Here's the drawing with two shaded views (mm, measured from the low corner). I have some questions. Coordinates: 2 decimals unless noted, no trailing zeros. Order: outer loops, then holes, each group sorted by start corner. A loop starts at its lowest first (then second) coordinate and runs counter-clockwise, first axis right, second up. Notation, with made-up numbers: (-19.75, -15.75) -> (-5.75, -15.75) arc R26 cw to (-5.75, 17.25) -> close; hole circle Ø5 at (74, 3.5). An arc over 180 degrees is marked (long way). Write item = value, one per line.
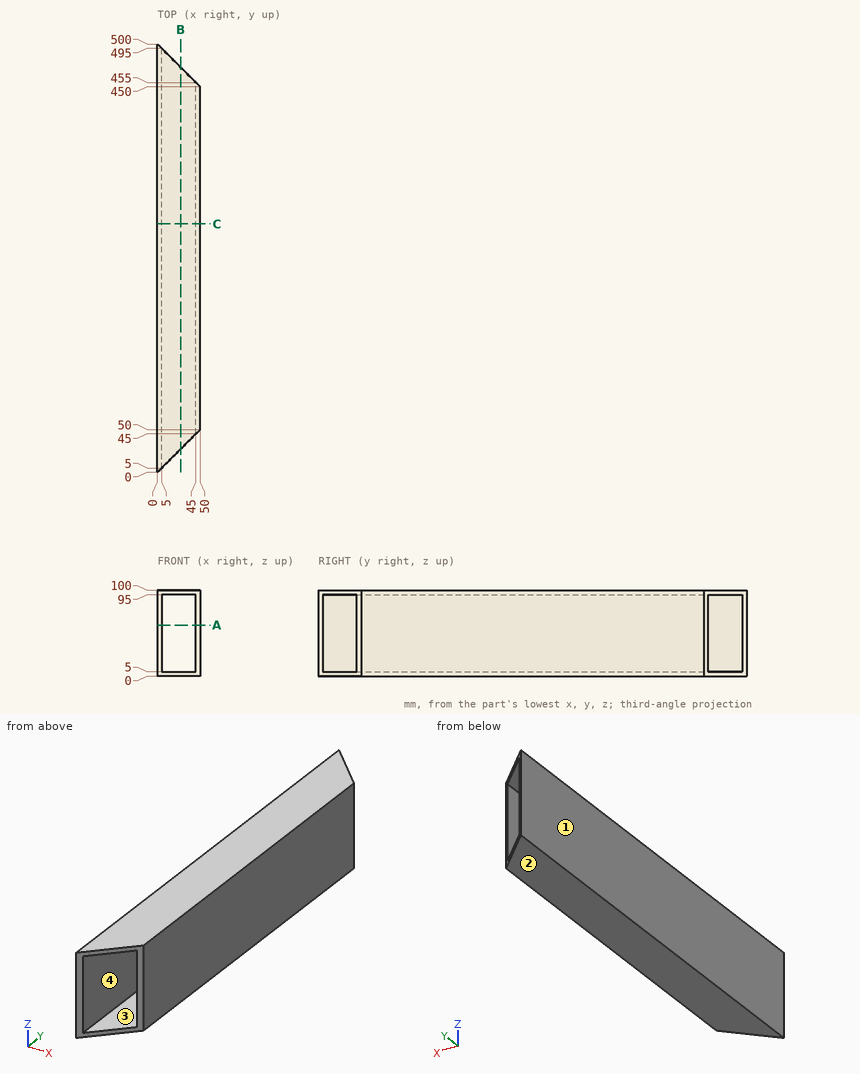
Item 1: I want a section at B-B, the plane x = 27. Please give me the cut outline in (y, z).
A:
outline = (27, 0) -> (473, 0) -> (473, 5) -> (27, 5) -> close; (27, 95) -> (473, 95) -> (473, 100) -> (27, 100) -> close
Item 2: I want a section at C-C, the plane y = 290. Please give me the cut outline in (x, z).
A:
outline = (0, 0) -> (50, 0) -> (50, 100) -> (0, 100) -> close; hole (5, 5) -> (45, 5) -> (45, 95) -> (5, 95) -> close
Item 3: I'm going to push flat-ended pins straight in: P1, Ø5, axis at x = 14, y = 93, coming from the -Z side; P2, Ø6, axis at x = 7.5, z = 54, coming from the -Y side. Where does each tip first touch, or does it pass through?
A:
P1 = 0
P2 = 4.5
Item 4: If we mould it in two halves opening along X, with no side actions, what happens to the marked faces 1, 2, 3 and 4? For each: pulls with the +X half, pulls with the -X half, needs draft (parallel to the pull), parting line crosses it, or undercut.
A:
face_1 = pulls with the -X half
face_2 = needs draft
face_3 = undercut
face_4 = undercut
Item 5: I want a section at A-A, the plane z = 59.5. Please give me the cut outline in (x, y), plus the area to 3 significant figures.
A:
outline = (0, 0) -> (5, 5) -> (5, 495) -> (0, 500) -> close; (45, 45) -> (50, 50) -> (50, 450) -> (45, 455) -> close
area = 4,500 mm2
Item 6: If I drill on probe 1 along Z at (x, y) = (25, 466); probe 2 along X at (y, z) = (342.5, 31.5); probe 3 along X at (y, z) = (42.5, 51.5), over which ranges is the centre line in solid material (lowest first)?
A:
probe_1 = 0 to 5, 95 to 100
probe_2 = 0 to 5, 45 to 50
probe_3 = 0 to 5
